Source: CAD feature listing. Evaluate the final solid. Frame: model axes, mm. A direction names the side the tool comes from. Give positions to 0.01 mm unless a question says otherwise; leave off trailing zeros. Loops run counter-clockwise (first coordinate to the right, second up) from the corner with the lowest first, then second, coordinate; pieces in that order, holes last.
```python
from build123d import *

# Parameters (mm, degrees)
SKETCH1_W           = 17
SKETCH1_H           = 17
BOSS_EXTRUDE1_DEPTH = 405
CUT_EXTRUDE2_DEPTH  = 406.986452976
CUT_EXTRUDE4_DEPTH  = 20
CUT_EXTRUDE5_DEPTH  = 406.986452976


with BuildPart() as part:
    # Sketch1 → Boss-Extrude1 (new body)
    with BuildSketch(Plane(origin=(0, 0, 0), x_dir=(1, 0, 0), z_dir=(0, 1, 0))):
        with BuildLine():
            Line((0.5, 0), (19.5, 0))
            ThreePointArc((19.5, 0), (19.853553391, 0.146446609), (20, 0.5))
            Line((20, 0.5), (20, 19.5))
            ThreePointArc((20, 19.5), (19.853553391, 19.853553391), (19.5, 20))
            Line((19.5, 20), (0.5, 20))
            ThreePointArc((0.5, 20), (0.146446609, 19.853553391), (0, 19.5))
            Line((0, 19.5), (0, 0.5))
            ThreePointArc((0, 0.5), (0.146446609, 0.146446609), (0.5, 0))
        make_face()
        with Locations((10, 10)):
            Rectangle(SKETCH1_W, SKETCH1_H, mode=Mode.SUBTRACT)
    extrude(amount=BOSS_EXTRUDE1_DEPTH)

    # Sketch4 → Cut-Extrude2 (cut, through all)
    with BuildSketch(Plane(origin=(0, 0, -20), x_dir=(-1, 0, 0), z_dir=(0, 0, -1))):
        Polygon((-5, 405), (-5, 395.773502692), (-15, 390), (-15, 405), align=None)
    extrude(amount=-CUT_EXTRUDE2_DEPTH, mode=Mode.SUBTRACT)

    # Sketch2 → Cut-Extrude4 (cut)
    with BuildSketch(Plane.XY):
        Polygon((20, 0), (20, 34.641016151), (0, 0), align=None)
    extrude(amount=-CUT_EXTRUDE4_DEPTH, mode=Mode.SUBTRACT)

    # Sketch6 → Cut-Extrude5 (cut, through all)
    with BuildSketch(Plane(origin=(0, 0, -20), x_dir=(-1, 0, 0), z_dir=(0, 0, -1))):
        Polygon((-2.59, 4.486011592), (-2.59, 24.486011592), (-10.09, 37.476392648), (-10.09, 17.476392648), align=None)
    extrude(amount=-CUT_EXTRUDE5_DEPTH, mode=Mode.SUBTRACT)


solid = part.part
```
(1) Mould query, pull axis X, two halves, no side actions, for faces 1 (the flat face through (6.288, 30.89, -0.761)), 2 (the flat face through (18.74, 32.46, -10.69)), 3 (the flat face through (0, 200, -10)). Classes: pulls with the +X half, pulls with the -X half, needs draft (parallel to the pull), parting line crosses it, or undercut.
A:
face 1: undercut
face 2: pulls with the +X half
face 3: pulls with the -X half
(2) First-contact query: pin 1 (0.8 mm diameter, centred on y = 13, z = -0.5, fed in from +X). Flat tip, straight axial feed; report the tip coordinate or a pass-through.
A:
pin 1: stops at x = 2.59
(3) Ray query, line 1 along Z through (x, y) = (15.5, 248.5); line 2 along X through (y, z) = (305, -8); line 3 along Y through (x, z) = (6.25, -1.25). Return the intervals inside material, ascending.
A:
line 1: z = -20 to -18.5, -1.5 to 0
line 2: x = 0 to 1.5, 18.5 to 20
line 3: y = 30.83 to 395.05
(4) Section B-B, the plane y = 192.5. Return the cut outline in (x, z).
A:
outline: (0, -19.5) arc R0.5 ccw to (0.5, -20) - (19.5, -20) arc R0.5 ccw to (20, -19.5) - (20, -0.5) arc R0.5 ccw to (19.5, 0) - (0.5, 0) arc R0.5 ccw to (0, -0.5) - close; hole (1.5, -18.5) - (18.5, -18.5) - (18.5, -1.5) - (1.5, -1.5) - close
(5) Reachability of faces 4 (the flat face through (20, 217, -10)), 5 (the flat face through (18.5, 216, -10)) from +Z, -Z, +X, -X, +Y, -Y: full face, straight path, thin tool, end or side. Return the list, or none.
A:
face 4: +Z, -Z, +X, +Y, -Y
face 5: +Y, -Y
(6) Section A-A, the plane z = -15. Return the cut outline in (x, y), then the cut area to 3 significant figures.
A:
outline: (0, 0) - (1.5, 2.6) - (1.5, 405) - (0, 405) - close; (18.5, 32.04) - (20, 34.64) - (20, 405) - (18.5, 405) - close
area: 1,160 mm2
(7) Section C-C, the plane y = 28.5. Return the cut outline in (x, z), then the cut area to 3 significant figures.
A:
outline: (0, -19.5) arc R0.5 ccw to (0.5, -20) - (4.91, -20) - (4.91, -18.5) - (1.5, -18.5) - (1.5, -1.5) - (4.91, -1.5) - (4.91, 0) - (0.5, 0) arc R0.5 ccw to (0, -0.5) - close; (10.09, -20) - (16.45, -20) - (16.45, -18.5) - (10.09, -18.5) - close; (10.09, -1.5) - (16.45, -1.5) - (16.45, 0) - (10.09, 0) - close
area: 59.2 mm2
